Here's how the part is built. I have some questions about the finished solid (model axes, mm). A direction names the side the tool comes from. Round coordinates to 2 decimals unless told otherwise and drop trailing zeros. Order: outer loops, then holes, each group sorted by start corner. A loop starts at its lowest first (then second) coordinate and runs counter-clockwise, first axis right, second up.
```python
from build123d import *

# Parameters (mm, degrees)
F0_W      = 63.6
F0_H      = 31.8
F1_DEPTH  = 9.6
F2_W      = 61.2
F2_H      = 29.4
F3_DEPTH  = 2
F4_R      = 2
F6_W      = 61.2
F6_H      = 29.4
F7_DEPTH  = 7.2
F8_R      = 3.25685
F10_DEPTH = 2.4
F9_R      = 2.4
F11_DEPTH = 2
F13_DEPTH = 32


with BuildPart() as f1:
    # F0 (on Top) → F1 (new body)
    with BuildSketch(Plane.XY):
        Rectangle(F0_W, F0_H)
    extrude(amount=F1_DEPTH)

    # F2 (on Top) → F3 (cut)
    with BuildSketch(Plane.XY):
        Rectangle(F2_W, F2_H)
    extrude(amount=F3_DEPTH, mode=Mode.SUBTRACT)

    # F4
    f4_edges = [f1.edges().sort_by_distance(p)[0] for p in [
        (-31.8, -15.9, 4.8),
        (-31.8, 15.9, 4.8),
        (31.8, 15.9, 4.8),
        (31.8, -15.9, 4.8),
    ]]
    fillet(f4_edges, radius=F4_R)

    # F6 (on offset) → F7 (cut)
    with BuildSketch(Plane.XY.offset(9.6)):
        Rectangle(F6_W, F6_H)
    extrude(amount=-F7_DEPTH, mode=Mode.SUBTRACT)

    # F8 (on Top) → F10 (join)
    with BuildSketch(Plane.XY):
        with Locations((-23.9, -8)):
            Circle(F8_R)
        with Locations((-23.9, 0)):
            Circle(F8_R)
        with Locations((-23.9, 8)):
            Circle(F8_R)
        with Locations((-15.900151, -7.950921)):
            Circle(F8_R)
        with Locations((-15.900151, 0.049079)):
            Circle(F8_R)
        with Locations((-15.900151, 8.049079)):
            Circle(F8_R)
        with Locations((-7.900301, -7.901842)):
            Circle(F8_R)
        with Locations((-7.900301, 0.098158)):
            Circle(F8_R)
        with Locations((-7.900301, 8.098158)):
            Circle(F8_R)
        with Locations((0.099548, -7.852764)):
            Circle(F8_R)
        with Locations((0.099548, 0.147236)):
            Circle(F8_R)
        with Locations((0.099548, 8.147236)):
            Circle(F8_R)
        with Locations((8.099398, -7.803685)):
            Circle(F8_R)
        with Locations((8.099398, 0.196315)):
            Circle(F8_R)
        with Locations((8.099398, 8.196315)):
            Circle(F8_R)
        with Locations((16.099247, -7.754606)):
            Circle(F8_R)
        with Locations((16.099247, 0.245394)):
            Circle(F8_R)
        with Locations((16.099247, 8.245394)):
            Circle(F8_R)
        with Locations((24.099097, -7.705527)):
            Circle(F8_R)
        with Locations((24.099097, 0.294473)):
            Circle(F8_R)
        with Locations((24.099097, 8.294473)):
            Circle(F8_R)
    extrude(amount=F10_DEPTH)

    # F9 (on Top) → F11 (cut)
    with BuildSketch(Plane.XY):
        with Locations((-23.9, -8)):
            Circle(F9_R)
        with Locations((-23.9, 0)):
            Circle(F9_R)
        with Locations((-23.9, 8)):
            Circle(F9_R)
        with Locations((-15.9, -8)):
            Circle(F9_R)
        with Locations((-15.9, 0)):
            Circle(F9_R)
        with Locations((-15.9, 8)):
            Circle(F9_R)
        with Locations((-7.9, -8)):
            Circle(F9_R)
        with Locations((-7.9, 0)):
            Circle(F9_R)
        with Locations((-7.9, 8)):
            Circle(F9_R)
        with Locations((0.1, -8)):
            Circle(F9_R)
        with Locations((0.1, 0)):
            Circle(F9_R)
        with Locations((0.1, 8)):
            Circle(F9_R)
        with Locations((8.1, -8)):
            Circle(F9_R)
        with Locations((8.1, 0)):
            Circle(F9_R)
        with Locations((8.1, 8)):
            Circle(F9_R)
        with Locations((16.1, -8)):
            Circle(F9_R)
        with Locations((16.1, 0)):
            Circle(F9_R)
        with Locations((16.1, 8)):
            Circle(F9_R)
        with Locations((24.1, -8)):
            Circle(F9_R)
        with Locations((24.1, 0)):
            Circle(F9_R)
        with Locations((24.1, 8)):
            Circle(F9_R)
    extrude(amount=F11_DEPTH, mode=Mode.SUBTRACT)

    # F12 (on Right) → F13 (cut)
    with BuildSketch(Plane.YZ):
        with BuildLine():
            Line((3.704295, 11.1), (-3.715705, 11.1))
            ThreePointArc((-3.715705, 11.1), (-4.352101, 10.836396), (-4.615705, 10.2))
            Line((-4.615705, 10.2), (-4.615705, 9))
            ThreePointArc((-4.615705, 9), (-4.352101, 8.363604), (-3.715705, 8.1))
            Line((-3.715705, 8.1), (3.704295, 8.1))
            ThreePointArc((3.704295, 8.1), (4.340691, 8.363604), (4.604295, 9))
            Line((4.604295, 9), (4.604295, 10.2))
            ThreePointArc((4.604295, 10.2), (4.340691, 10.836396), (3.704295, 11.1))
        make_face()
    extrude(amount=F13_DEPTH, mode=Mode.SUBTRACT)


solid = f1.part
```
1. If we section it at D-D, the plane z = 1: State how many separate pieces and enclosed holes the cut face has, and give its area (3 significant figures).
Evaluation:
separate pieces: 22
enclosed holes: 22
area: 540 mm2
2. On a 3-axis mill with a long thin cutter (end or side, diameter ignored), from which of +Z, -Z, +X, -X, +Y, -Y can I reach the whole of each face in a straight line? I mean faces 5 (the flat face through (-10, -15, 9.6)), 6 (the flat face through (16, -8, 2)). Say none if no direction works.
Evaluation:
face 5: +Z, +X, -X, +Y, -Y
face 6: -Z
3. If we section it at B-B, the plane x = 20: Write out the boundary of the cut face in (y, z).
Evaluation:
outline: (-15.9, 0) - (-14.7, 0) - (-14.7, 2) - (14.7, 2) - (14.7, 0) - (15.9, 0) - (15.9, 9.6) - (14.7, 9.6) - (14.7, 2.4) - (-14.7, 2.4) - (-14.7, 9.6) - (-15.9, 9.6) - close
4. If we mould it in two halves opening along X, with no side actions, what happens to faces 1 (the flat face through (2, -10, 0)), 2 (the cylindrical face through (-0.324, -4.624, 0.986)), 3 (the cylindrical face through (-13.61, 8.72, 0.99)), 4 (the cylindrical face through (31.2, 15.33, 4.87))? For each: released by +X, released by -X, zero draft, split by the parting line, or undercut.
Evaluation:
face 1: zero draft
face 2: undercut
face 3: undercut
face 4: released by +X
5. I'm going to push flat-ended pins straight in: P1, Ø1, axis at x = -2, y = 9.5, coming from the -Z side; P2, Ø7.5, axis at x = -7.9, y = -8, coming from the +Z side; P3, Ø3, axis at x = 16.1, y = 0, coming from the -Z side. Where does each tip first touch, or does it pass through?
Evaluation:
P1: stops at z = 0
P2: stops at z = 2.4
P3: stops at z = 2
6. If we section it at A-A, the plane z = 5.5: Write out the boundary of the cut face in (x, y).
Evaluation:
outline: (-31.8, -13.9) arc R2 ccw to (-29.8, -15.9) - (29.8, -15.9) arc R2 ccw to (31.8, -13.9) - (31.8, 13.9) arc R2 ccw to (29.8, 15.9) - (-29.8, 15.9) arc R2 ccw to (-31.8, 13.9) - close; hole (-30.6, -14.7) - (30.6, -14.7) - (30.6, 14.7) - (-30.6, 14.7) - close
7. If we section it at C-C, the plane y = -12: Write out the boundary of the cut face in (x, z), and give its area (3 significant figures).
Evaluation:
outline: (-31.8, 0) - (-30.6, 0) - (-30.6, 2) - (30.6, 2) - (30.6, 0) - (31.8, 0) - (31.8, 9.6) - (30.6, 9.6) - (30.6, 2.4) - (-30.6, 2.4) - (-30.6, 9.6) - (-31.8, 9.6) - close
area: 47.5 mm2
8. I need wall thicknesses on probe 1 along Y at (x, z) = (-8, 9.25); probe 2 along X at (y, z) = (10, 9.25); probe 3 along Z at (x, y) = (-15.5, 6). Which ranges of each line are inside material? Lowest first, please.
Evaluation:
probe 1: y = -15.9 to -14.7, 14.7 to 15.9
probe 2: x = -31.8 to -30.6, 30.6 to 31.8
probe 3: z = 2 to 2.4
